For this review, take the finished solid that the model builds, in its own axes (mm). A direction names the side the tool comes from. Give positions to 0.01 mm unless a question says otherwise; leave off trailing zeros. Order: outer loops, then holes, each group sorted by start corner. A loop starts at its lowest first (then second) coordinate and runs counter-clockwise, first axis right, second up. Notation, with made-up numbers: (47.25, 76) - (75.25, 76) arc R21 ccw to (75.25, 111) - close; hole circle Ø5 at (-7.75, 33). An arc over 180 degrees is marked (long way). One line per item, written item: value.
```python
from build123d import *

# Parameters (mm, degrees)
SKETCH_R     = 2.2
PAD_DEPTH    = 3
POCKET_DEPTH = 2


with BuildPart() as part:
    # Sketch → Pad (new body)
    with BuildSketch(Plane.XY):
        Polygon((6.470319, -4.525), (-6.470319, -4.525), (-6.470319, 0.643078), (-3.4208, 5.925), (3.4208, 5.925), (6.470319, 0.643078), align=None)
        Circle(SKETCH_R, mode=Mode.SUBTRACT)
    extrude(amount=PAD_DEPTH)

    # Sketch001 → Pocket (cut)
    with BuildSketch(Plane.XY.offset(3)):
        Polygon((4.070319, 0), (2.03516, 3.525), (-2.03516, 3.525), (-4.070319, 0), (-2.03516, -3.525), (2.03516, -3.525), align=None)
    extrude(amount=-POCKET_DEPTH, mode=Mode.SUBTRACT)


solid = part.part
```
(1) Take a section at A-A (z = 0.2). Write out the cut boundary in (x, y) (3 decimals), then the cut area to 3 significant figures.
Answers below:
outline: (-6.47, -4.525) - (6.47, -4.525) - (6.47, 0.643) - (3.421, 5.925) - (-3.421, 5.925) - (-6.47, 0.643) - close; hole circle Ø4.4 at (0, 0)
area: 104 mm^2
(2) Draft analysis for pull direction Y (two halves, no side actions). For faces 3 (the face through (-6.47, -2, 1)), 4 (the face through (3.067, 1.738, 2.014)), 5 (the face through (-4.967, 3.247, 1.479)), state which applies: pulls with the +Y half, pulls with the -Y half, needs draft (parallel to the pull), parting line crosses it, or undercut.
Answers below:
face 3: needs draft
face 4: undercut
face 5: pulls with the +Y half
(3) For P1, Ø5, axis at x = 0, y = 0, coming from the -Z side, flat-tipped, find the tip position at first contact; note if it passes through.
Answers below:
P1: stops at z = 0
(4) Take a section at B-B (y = -1.75). Write out the cut boundary in (x, z), then the cut area to 3 significant figures.
Answers below:
outline: (-6.47, 0) - (-1.33, 0) - (-1.33, 1) - (-3.06, 1) - (-3.06, 3) - (-6.47, 3) - close; (1.33, 0) - (6.47, 0) - (6.47, 3) - (3.06, 3) - (3.06, 1) - (1.33, 1) - close
area: 23.9 mm^2
(5) Machinability: for faces 1 (the face through (2, 2, 1)), 2 (the face through (6.47, -2, 1)), which of the approach directions +Z, -Z, +X, -X, +Y, -Y give a long, thin tool a straight path to every point of the face, cutting with its end or side? Answer none if there is none.
Answers below:
face 1: +Z
face 2: +Z, -Z, +X, +Y, -Y
(6) Wall thickness on line 1 (X direction, y = 0, z = 0.6); line 2 (Y direction, x = 0, z = 0.35) (3 decimals); line 3 (Y direction, x = 1, z = 1.15) (3 decimals): over which ranges is each line inside the solid? List them lowest first. Write a range as from..to.
Answers below:
line 1: x = -6.47..-2.2, 2.2..6.47
line 2: y = -4.525..-2.2, 2.2..5.925
line 3: y = -4.525..-3.525, 3.525..5.925
(7) Take a section at D-D (z = 1.35). Write out the cut boundary in (x, y) (3 decimals).
Answers below:
outline: (-6.47, -4.525) - (6.47, -4.525) - (6.47, 0.643) - (3.421, 5.925) - (-3.421, 5.925) - (-6.47, 0.643) - close; hole (-4.07, 0) - (-2.035, -3.525) - (2.035, -3.525) - (4.07, 0) - (2.035, 3.525) - (-2.035, 3.525) - close
(8) Take a section at C-C (x = 0). Write out the cut boundary in (y, z) (3 decimals).
Answers below:
outline: (-4.525, 0) - (-2.2, 0) - (-2.2, 1) - (-3.525, 1) - (-3.525, 3) - (-4.525, 3) - close; (2.2, 0) - (5.925, 0) - (5.925, 3) - (3.525, 3) - (3.525, 1) - (2.2, 1) - close
